Check sheet for the modelled part. Datum: model origin and axes. Units: mm. Round coordinates to 2 decimals unless told otherwise and drop trailing zeros. Loops run counter-clockwise (first coordinate to the right, second up) from the corner with the lowest first, then second, coordinate; pieces in that order, holes last. Notation, with made-up numbers: (-1.75, -1) -> (8.25, -1) arc R16 cw to (8.25, 19) -> close; hole circle Ø6 at (24.25, 87). An arc over 180 degrees is marked (long way). Use one line per item in the form item = value. Start each with the question number.
(1) Material ranges on probe 1 along X at (y, z) = (19, 0.7); probe 2 along X at (y, z) = (15.75, 2); probe 3 along Y at (x, z) = (-29, 2.3), recorded low to high. Write a range as [from, to].
(2) Sectioned sample at C-C (z = 1.3). Record the cut outline in (x, y).
(3) Sectioned sample at D-D (y = 24.25). Record the cut outline in (x, z), and give its area (3 significant figures).
(4) Sectioned sample at A-A (y = 21.75). Record the cut outline in (x, z), and give its area (3 significant figures).
(5) Sectioned sample at B-B (x = -25). Record the cut outline in (y, z), and give its area (3 significant figures).
(6) Draft check along Y on faces 1 (the cylindrical face through (-48.3, 25.83, 1.52)), 2 (the cylindrical face through (-14.55, 26.19, 1.52)), 3 (the cylindrical face through (-50.89, 26.72, 1.52)), 4 (the flat face through (-32, 10.219, 1)). Enter one of: released by +Y, released by -Y, zero draft, split by the parting line, or undercut.
(7) Go/stop test with a flat-tipped pin: pin 1 (1 mm diameter, centred on y = 14, z = 1.5, fed in from +X). Record where the tip stops, or that it passes through.
from build123d import *

# Parameters (mm, degrees)
F0_W     = 42
F0_H     = 18
F1_DEPTH = 3
F2_D     = 3.2
F3_D     = 8
F4_R     = 5


with BuildPart() as f1:
    # F0 (on Top) → F1 (new body)
    with BuildSketch(Plane.XY):
        with Locations((-31.3194459304, 19.2188901754)):
            Rectangle(F0_W, F0_H)
    extrude(amount=F1_DEPTH)

    # F2 (through all)
    with Locations(Plane(origin=(0, 0, 0), x_dir=(1, 0, 0), z_dir=(0, 0, -1))):
        with Locations((-46.8194459304, -25.2188901754), (-15.8194459304, -25.2188901754)):
            Hole(F2_D / 2)

    # F3 (through all)
    with Locations(Plane(origin=(0, 0, 0), x_dir=(1, 0, 0), z_dir=(0, 0, -1))):
        with Locations((-25.3194459304, -19.2188901754), (-37.3194459304, -19.2188901754)):
            Hole(F3_D / 2)

    # F4
    f4_edges = [f1.edges().sort_by_distance(p)[0] for p in [
        (-52.319446, 28.21889, 1.5),
        (-52.319446, 10.21889, 1.5),
        (-10.319446, 28.21889, 1.5),
        (-10.319446, 10.21889, 1.5),
    ]]
    fillet(f4_edges, radius=F4_R)


solid = f1.part
Checks:
q1.probe_1 = [-52.32, -41.31], [-33.33, -29.31], [-21.33, -10.32]
q1.probe_2 = [-52.32, -39.31], [-35.33, -27.31], [-23.33, -10.32]
q1.probe_3 = [10.22, 17.65], [20.79, 28.22]
q2.outline = (-52.32, 15.22) arc R5 ccw to (-47.32, 10.22) -> (-15.32, 10.22) arc R5 ccw to (-10.32, 15.22) -> (-10.32, 23.22) arc R5 ccw to (-15.32, 28.22) -> (-47.32, 28.22) arc R5 ccw to (-52.32, 23.22) -> close; hole circle Ø3.2 at (-46.82, 25.22); hole circle Ø8 at (-37.32, 19.22); hole circle Ø8 at (-25.32, 19.22); hole circle Ø3.2 at (-15.82, 25.22)
q3.outline = (-52.21, 0) -> (-48.09, 0) -> (-48.09, 3) -> (-52.21, 3) -> close; (-45.55, 0) -> (-17.09, 0) -> (-17.09, 3) -> (-45.55, 3) -> close; (-14.55, 0) -> (-10.43, 0) -> (-10.43, 3) -> (-14.55, 3) -> close
q3.area = 110 mm2
q4.outline = (-52.32, 0) -> (-40.42, 0) -> (-40.42, 3) -> (-52.32, 3) -> close; (-34.22, 0) -> (-28.42, 0) -> (-28.42, 3) -> (-34.22, 3) -> close; (-22.22, 0) -> (-10.32, 0) -> (-10.32, 3) -> (-22.22, 3) -> close
q4.area = 88.8 mm2
q5.outline = (10.22, 0) -> (15.23, 0) -> (15.23, 3) -> (10.22, 3) -> close; (23.21, 0) -> (28.22, 0) -> (28.22, 3) -> (23.21, 3) -> close
q5.area = 30.1 mm2
q6.face_1 = undercut
q6.face_2 = undercut
q6.face_3 = released by +Y
q6.face_4 = released by -Y
q7.pin_1 = -10.37
